from build123d import *

# Parameters (mm, degrees)
F0_R     = 1.524
F0_R_2   = 1.04775
F0_W     = 12.4206
F0_H     = 22.5806
F1_DEPTH = 3.175


# Not quite as in the source:
# - ends of sketch curves that miss each other by under 0.0002 mm in the source are joined
# - a length typed as a fraction of an inch, garbled in the dataset ("3 / 203.2 mm" for 3/8 in), is restored


with BuildPart() as f1:
    # F0 (on Top) → F1 (new body)
    with BuildSketch(Plane.XY):
        with BuildLine():
            ThreePointArc((19.0496193061, 35.359281088), (17.1886928512, 39.8489739211), (12.6981263868, 41.7077912426))
            Line((12.6981263868, 41.7077912426), (-12.7018729111, 41.7018188664))
            ThreePointArc((-12.7018729111, 41.7018188664), (-17.19156232, 39.8408924124), (-19.0503796423, 35.3503293721))
            Line((-19.0503796423, 35.3503293721), (-19.0399523971, -9.0977780687))
            Line((-19.0399523971, -9.0977780687), (-10.8996863639, -9.0977780687))
            Line((-10.8996863639, -9.0977780687), (-10.8996863639, -12.2727780687))
            Line((-10.8996863639, -12.2727780687), (-14.0746863639, -12.2727780687))
            Line((-14.0746863639, -12.2727780687), (-14.0746863639, -18.6227780687))
            Line((-14.0746863639, -18.6227780687), (-10.8996939729, -18.6227780687))
            Line((-10.8996939729, -18.6227780687), (-10.8996939729, -26.3697780687))
            Line((-10.8996939729, -26.3697780687), (-7.8538059598, -26.3697780687))
            Line((-7.8538059598, -26.3697780687), (-7.8538059598, -24.2107780687))
            Line((-7.8538059598, -24.2107780687), (-4.8058059598, -24.2107780687))
            Line((-4.8058059598, -24.2107780687), (-4.8058059598, -26.3697780687))
            Line((-4.8058059598, -26.3697780687), (-2.0297826182, -26.3697780687))
            Line((-2.0297826182, -26.3697780687), (-2.0297826182, -29.9257780687))
            Line((-2.0297826182, -29.9257780687), (-4.8058059598, -29.9257780687))
            Line((-4.8058059598, -29.9257780687), (-4.8058059598, -32.0847780687))
            Line((-4.8058059598, -32.0847780687), (-7.8538059598, -32.0847780687))
            Line((-7.8538059598, -32.0847780687), (-7.8538059598, -29.9257780687))
            Line((-7.8538059598, -29.9257780687), (-10.8996939729, -29.9257780687))
            Line((-10.8996939729, -29.9257780687), (-10.8996939729, -34.4977780687))
            Line((-10.8996939729, -34.4977780687), (10.9197826182, -34.4977780687))
            Line((10.9197826182, -34.4977780687), (10.9197826182, -29.9257780687))
            Line((10.9197826182, -29.9257780687), (7.8538059598, -29.9257780687))
            Line((7.8538059598, -29.9257780687), (7.8538059598, -32.0847780687))
            Line((7.8538059598, -32.0847780687), (4.8058059598, -32.0847780687))
            Line((4.8058059598, -32.0847780687), (4.8058059598, -29.9257780687))
            Line((4.8058059598, -29.9257780687), (2.0297826182, -29.9257780687))
            Line((2.0297826182, -29.9257780687), (2.0297826182, -26.3697780687))
            Line((2.0297826182, -26.3697780687), (4.8058059598, -26.3697780687))
            Line((4.8058059598, -26.3697780687), (4.8058059598, -24.2107780687))
            Line((4.8058059598, -24.2107780687), (7.8538059598, -24.2107780687))
            Line((7.8538059598, -24.2107780687), (7.8538059598, -26.3697780687))
            Line((7.8538059598, -26.3697780687), (10.9197826182, -26.3697780687))
            Line((10.9197826182, -26.3697780687), (10.9197826182, -18.6227780687))
            Line((10.9197826182, -18.6227780687), (14.0947826182, -18.6227780687))
            Line((14.0947826182, -18.6227780687), (14.0947826182, -12.2727780687))
            Line((14.0947826182, -12.2727780687), (10.9197826182, -12.2727780687))
            Line((10.9197826182, -12.2727780687), (10.9197826182, -9.0977780687))
            Line((10.9197826182, -9.0977780687), (19.0600486513, -9.0977780687))
            Line((19.0600486513, -9.0977780687), (19.0496193061, 35.359281088))
        make_face()
        with Locations((-7.0950099938, 1.5702219313)):
            Circle(F0_R, mode=Mode.SUBTRACT)
        with Locations((7.0950099938, -6.8244780687)):
            Circle(F0_R_2, mode=Mode.SUBTRACT)
        with Locations((-7.0950099938, 37.1302219313)):
            Circle(F0_R, mode=Mode.SUBTRACT)
        with Locations((7.0950099938, 7.1455219313)):
            Rectangle(F0_W, F0_H, mode=Mode.SUBTRACT)
        with Locations((7.0950099938, 21.1155219313)):
            Circle(F0_R_2, mode=Mode.SUBTRACT)
        with Locations((7.0950099938, 37.1302219313)):
            Circle(F0_R, mode=Mode.SUBTRACT)
    extrude(amount=F1_DEPTH)


solid = f1.part
Source: CAD feature listing. Evaluate the final solid. Frame: model axes, mm. A direction names the side the tool comes from. Coordinates: 2 decimals unless noted, no trailing zeros. Loops run counter-clockwise (first coordinate to the right, second up) from the corner with the lowest first, then second, coordinate; pieces in that order, holes last. Notation, with made-up numbers: M -40,84.25 L -29,84.25 A33 cw -29,123.25 Z; hole C -9,1.5 d2. An arc over 180 degrees is marked long. Answer in a Markdown table with one row per item.
Q1. Set-up query: faces 1 (the flat face through (7.854, -31, 2)), 2 (the flat face through (-9, -26.37, 2)), 3 (the flat face through (13, -12.273, 2)). Return all of +Z, -Z, +X, -X, +Y, -Y with unobstructed straight access to the full face (end or side cutting, diameter ignored); none if empty.
Answers below:
| item | result |
|---|---|
| face 1 | +Z, -Z |
| face 2 | +Z, -Z, -X |
| face 3 | +Z, -Z, +X |
Q2. Section C-C on y = -2. Return the cut outline in (x, z) (3 decimals), plus the area to 3 significant figures.
Answers below:
| item | result |
|---|---|
| outline | M -19.042,0 L 0.885,0 L 0.885,3.175 L -19.042,3.175 Z; M 13.305,0 L 19.058,0 L 19.058,3.175 L 13.305,3.175 Z |
| area | 81.5 mm^2 |
Q3. Draft query along Y for faces 4 (the flat face through (-10.9, -32, 2)), 5 (the flat face through (9, -26.37, 2)). Return one class per face: pulls with the +Y half, pulls with the -Y half, needs draft (parallel to the pull), parting line crosses it, or undercut.
Answers below:
| item | result |
|---|---|
| face 4 | needs draft |
| face 5 | undercut |
Q4. Section B-B on x = 12. Return the cut outline in (y, z) (3 decimals).
Answers below:
| item | result |
|---|---|
| outline | M -18.623,0 L -12.273,0 L -12.273,3.175 L -18.623,3.175 Z; M -9.098,0 L -4.145,0 L -4.145,3.175 L -9.098,3.175 Z; M 18.436,0 L 41.708,0 L 41.708,3.175 L 18.436,3.175 Z |
Q5. Section D-D on x = -4. Return the cut outline in (y, z) (3 decimals), plus the area to 3 significant figures.
Answers below:
| item | result |
|---|---|
| outline | M -34.498,0 L -29.926,0 L -29.926,3.175 L -34.498,3.175 Z; M -26.37,0 L 41.704,0 L 41.704,3.175 L -26.37,3.175 Z |
| area | 231 mm^2 |
Q6. Section A-A on y = -25. Return the cut outline in (x, z) (3 decimals), plus the area to 3 significant figures.
Answers below:
| item | result |
|---|---|
| outline | M -10.9,0 L -7.854,0 L -7.854,3.175 L -10.9,3.175 Z; M -4.806,0 L 4.806,0 L 4.806,3.175 L -4.806,3.175 Z; M 7.854,0 L 10.92,0 L 10.92,3.175 L 7.854,3.175 Z |
| area | 49.9 mm^2 |
Q7. First-contact query: pin 1 (1.1 mm diameter, centred on y = -31, z = 1, fed in from +X); pin 2 (1.5 mm diameter, centred on y = -12, z = 0.5, fed in from -X); pin 3 (1.5 mm diameter, centred on x = -8.5, z = 1, fed in from +Y). Flat tips, straight axial feed; report the tip coordinate or a pass-through.
Answers below:
| item | result |
|---|---|
| pin 1 | stops at x = 10.92 |
| pin 2 | stops at x = -14.07 |
| pin 3 | stops at y = 41.7 |
Q8. Ray query, probe 1 along Y at (x, z) = (12, 0.2); probe 2 along X at (y, z) = (-24.5, 2.6); probe 3 along Y at (x, z) = (9, 2.1). Return the intervals inside material, ascending. Write a range as from..to.
Answers below:
| item | result |
|---|---|
| probe 1 | y = -18.62..-12.27, -9.1..-4.14, 18.44..41.71 |
| probe 2 | x = -10.9..-7.85, -4.81..4.81, 7.85..10.92 |
| probe 3 | y = -34.5..-29.93, -26.37..-4.14, 18.44..41.71 |
